```python
from build123d import *

# Parameters (mm, degrees)
BOSS_EXTRUDE1_DEPTH = 3
BOSS_EXTRUDE2_DEPTH = 1.5
FILLET1_R           = 1
CUT_EXTRUDE1_REACH  = 25.5
SKETCH3_R           = 0.5


with BuildPart() as part:
    # Sketch1 → Boss-Extrude1 (new body)
    with BuildSketch(Plane(origin=(0, 0, 0), x_dir=(1, 0, 0), z_dir=(0, 1, 0))):
        with BuildLine():
            Line((3, -23.307724042), (3, -21.289668856))
            ThreePointArc((3, -21.289668856), (0, -21.5), (-3, -21.289668856))
            Line((-3, -21.289668856), (-3, -23.307724042))
            ThreePointArc((-3, -23.307724042), (0, -23.5), (3, -23.307724042))
        make_face()
    extrude(amount=BOSS_EXTRUDE1_DEPTH)

    # Sketch2 → Boss-Extrude2 (add)
    with BuildSketch(Plane(origin=(0, 3, 0), x_dir=(1, 0, 0), z_dir=(0, 1, 0))):
        with BuildLine():
            Line((-6, -22.721135535), (-6, -20.645822822))
            ThreePointArc((-6, -20.645822822), (0, -21.5), (6, -20.645822822))
            Line((6, -20.645822822), (6, -22.721135535))
            ThreePointArc((6, -22.721135535), (0, -23.5), (-6, -22.721135535))
        make_face()
    extrude(amount=-BOSS_EXTRUDE2_DEPTH)

    # Fillet1
    fillet1_edges = [part.edges().sort_by_distance(p)[0] for p in [
        (0, 3, 23.5),
    ]]
    fillet(fillet1_edges, radius=FILLET1_R)

    # Sketch3 → Cut-Extrude1 (cut, up to next)
    with BuildSketch(Plane.XY, mode=Mode.PRIVATE) as cut_extrude1_sk1:
        with Locations((0, 2)):
            Circle(SKETCH3_R)
    cut_extrude1_tool1 = extrude(cut_extrude1_sk1.sketch, amount=CUT_EXTRUDE1_REACH, mode=Mode.PRIVATE) & part.part
    add(cut_extrude1_tool1.solids().sort_by_distance((0, 2, 0))[0], mode=Mode.SUBTRACT)


solid = part.part
```
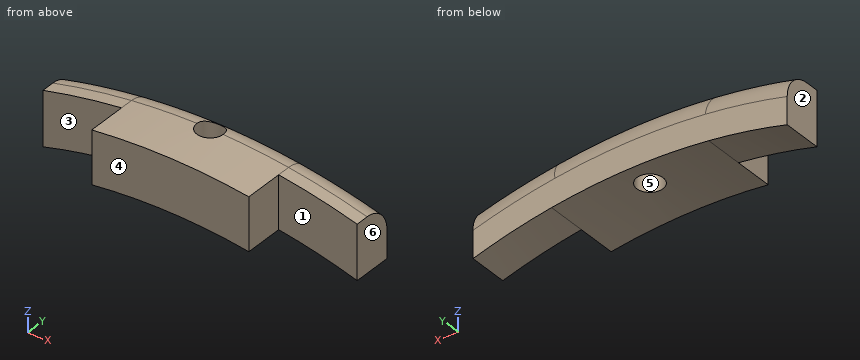
For this review, take the finished solid that the model builds, in its own axes (mm). Face numbers are marked on the shaded views. A direction names the side the tool comes from. Coordinates: 2 decimals unless noted, no trailing zeros. Loops run counter-clockwise (first coordinate to the right, second up) from the corner with the lowest first, then second, coordinate; pieces in that order, holes last.
1. Add section A-A, the plane y = 1.7. Give the boundary of the cut face in (x, z).
2. For line 1 (X direction, y = 2, z = 22.55); line 2 (Y direction, x = 0, z = 22.55); line 3 (Z direction, x = 3, y = 2), list the stretches that pass through material, from the lowest coordinate up.
3. For the marked faces 1, 2 and 3, list the 3-axis set-ups (+Z, -Z, +X, -X, +Y, -Y) from which the entire face can be reached by the end or side of a thin tool; tool diameter is ignored.
4. Add section C-C, the plane y = 0.5. Give the boundary of the cut face in (x, z), then the cut area to 3 significant figures.
5. Insertion check: P1, Ø1.3, axis at x = -4.5, z = 22, coming from the -Y side; P2, Ø0.8, axis at y = 1, z = 22, coming from the -X side. Each pin has a flat end and moves straight along its axis. Give the tip position at first contact, or say it passes through.
6. Mouldability with a two-part tool opening along Y and no side actions: class the marked faces 4, 5 and 6 as +Y half, -Y half, draft (parallel to the pull), parting line (faces both ways), or undercut.
7. Add section B-B, the plane x = 0. Give the boundary of the cut face in (y, z), then the cut area to 3 significant figures.
Result:
1. outline: (-6, 20.65) arc R21.5 cw to (-0.4, 21.5) - (-0.4, 23.5) arc R23.5 ccw to (-6, 22.72) - close; (0.4, 21.5) arc R21.5 cw to (6, 20.65) - (6, 22.72) arc R23.5 ccw to (0.4, 23.5) - close
2. line 1: x = -6 to -0.5, 0.5 to 6
2. line 2: y = 0 to 1.5, 2.5 to 3
2. line 3: z = 21.29 to 23.31
3. face 1: +Z, -Z, +X, -Y
3. face 2: +Z, -Z, -X, +Y, -Y
3. face 3: +Z, -Z, -X, -Y
4. outline: (-3, 21.29) arc R21.5 cw to (3, 21.29) - (3, 23.31) arc R23.5 ccw to (-3, 23.31) - close
4. area: 12.0 mm2
5. P1: stops at y = 1.5
5. P2: stops at x = -3
6. face 4: -Y half
6. face 5: undercut
6. face 6: draft
7. outline: (0, 21.5) - (1.5, 21.5) - (1.5, 23.5) - (0, 23.5) - close; (2.5, 21.5) - (3, 21.5) - (3, 22.5) arc R1 ccw to (2.5, 23.37) - close
7. area: 3.81 mm2
